```python
from build123d import *

# Parameters (mm, degrees)
SKETCH1_W                = 50
SKETCH1_H                = 40
BOSS_EXTRUDE1_DEPTH      = 20
SKETCH2_W                = 36
SKETCH2_H                = 16
CUT_EXTRUDE1_DEPTH       = 50
CUT_EXTRUDE2_REACH       = 53.235
BOSS_EXTRUDE2_DEPTH      = 5
BOSS_EXTRUDE2_DEPTH_BACK = 25
SKETCH5_R                = 9
BOSS_EXTRUDE3_START      = -19
SKETCH8_R                = 9
BOSS_EXTRUDE3_DEPTH      = 19
SKETCH9_R                = 8
CUT_EXTRUDE4_DEPTH       = 30


with BuildPart() as part:
    # Sketch1 → Boss-Extrude1 (new body)
    with BuildSketch(Plane(origin=(0, 0, 0), x_dir=(1, 0, 0), z_dir=(0, 1, 0))):
        Rectangle(SKETCH1_W, SKETCH1_H)
    extrude(amount=BOSS_EXTRUDE1_DEPTH)

    # Sketch2 → Cut-Extrude1 (cut)
    with BuildSketch(Plane(origin=(25, 0, 0), x_dir=(0, 0, -1), z_dir=(1, 0, 0))):
        with Locations((0, 10)):
            Rectangle(SKETCH2_W, SKETCH2_H)
    extrude(amount=-CUT_EXTRUDE1_DEPTH, mode=Mode.SUBTRACT)

    # Cut-Extrude2: up to this face of the body (flat: up to its plane)
    cut_extrude2_end = Plane(part.part.faces().sort_by_distance((0, 10, -20))[0])
    # Sketch3 → Cut-Extrude2 (cut, up to the picked face)
    with BuildSketch(Plane.XY.offset(20), mode=Mode.PRIVATE) as cut_extrude2_sk1:
        Polygon((25, 0), (25, 20), (10, 0), align=None)
    cut_extrude2_tool1 = split(extrude(cut_extrude2_sk1.sketch, amount=-CUT_EXTRUDE2_REACH, mode=Mode.PRIVATE), bisect_by=cut_extrude2_end, keep=Keep.BOTH, mode=Mode.PRIVATE)
    # Sketch3 → Cut-Extrude2 (cut, up to the picked face)
    with BuildSketch(Plane.XY.offset(20), mode=Mode.PRIVATE) as cut_extrude2_sk2:
        Polygon((-10, 0), (-25, 20), (-25, 0), align=None)
    cut_extrude2_tool2 = split(extrude(cut_extrude2_sk2.sketch, amount=-CUT_EXTRUDE2_REACH, mode=Mode.PRIVATE), bisect_by=cut_extrude2_end, keep=Keep.BOTH, mode=Mode.PRIVATE)
    add(cut_extrude2_tool1.solids().sort_by(Axis((20, 6.666667, 20), (0, 0, -1)))[0], mode=Mode.SUBTRACT)
    add(cut_extrude2_tool2.solids().sort_by(Axis((-20, 6.666667, 20), (0, 0, -1)))[0], mode=Mode.SUBTRACT)

    # Sketch5 → Boss-Extrude2 (add, two sides: drawn at the far end of the back side and taken through both)
    with BuildSketch(Plane(origin=(0, 20, 0), x_dir=(1, 0, 0), z_dir=(0, 1, 0)).offset(-BOSS_EXTRUDE2_DEPTH_BACK)):
        with Locations(Location((0, 0, 0), (0, 0, 90))):
            Circle(SKETCH5_R)
    extrude(amount=BOSS_EXTRUDE2_DEPTH + BOSS_EXTRUDE2_DEPTH_BACK)

    # Sketch8 → Boss-Extrude3 (add)
    with BuildSketch(Plane(origin=(0, -5, 0), x_dir=(-1, 0, 0), z_dir=(0, -1, 0)).offset(BOSS_EXTRUDE3_START)):
        with Locations(Location((0, 0, 0), (0, 0, 90))):
            Circle(SKETCH8_R)
    extrude(amount=BOSS_EXTRUDE3_DEPTH)

    # Sketch9 → Cut-Extrude4 (cut)
    with BuildSketch(Plane(origin=(0, 25, 0), x_dir=(1, 0, 0), z_dir=(0, 1, 0))):
        with Locations(Location((0, 0, 0), (0, 0, 270))):
            Circle(SKETCH9_R)
    extrude(amount=-CUT_EXTRUDE4_DEPTH, mode=Mode.SUBTRACT)


solid = part.part
```
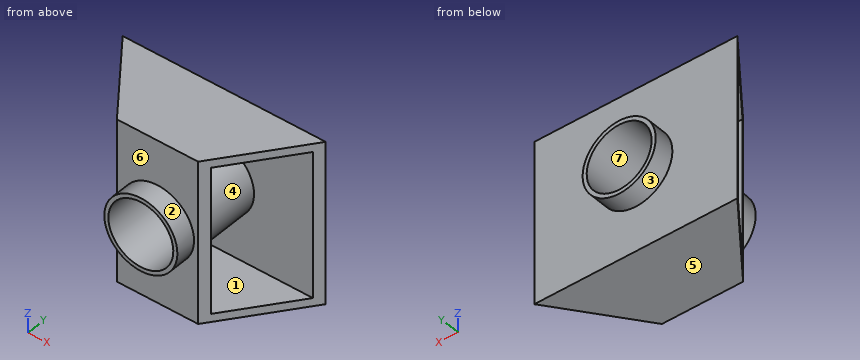
CAD build for the part. Positions are in the model's coordinates, mm. Face numbers are marked on the shaded views. A direction names the side the tool comes from. Coordinates: 2 decimals unless noted, no trailing zeros. Write each loop counter-clockwise with the first axis right and the second up, starting at its lowest first coordinate (ties: lowest second). Pieces come first, ordered by that corner, then holes. Notation, with made-up numbers: (13, -15) -> (72, -15) arc R9 cw to (72, -7) -> close; hole circle Ø2 at (-37, 4.5). An arc over 180 degrees is marked (long way). Use CSV: the item, a comma, the result in double quotes. Start each with the question number.
Item 1: Band-saw the part on B-B, the plane y = 11.25. Write the cut outline in (x, z).
Item 2: Two-plate mould, pull along Z, no slides. Class the marked faces 4, 5, 6 and 7: +Z half, -Z half, draft (parallel to the pull), parting line (faces both ways), or undercut.
Item 3: Band-saw the part on C-C, the plane z = 13.5. Write the cut outline in (x, y), plus the area to 3 significant figures.
Item 4: Band-saw the part on D-D, the plane y = 22.25. Write the cut outline in (x, z).
Item 5: Tool access for the marked faces 1, 2 and 3: list every direction of +Z, -Z, +X, -X, +Y, -Y with a clear straight run to the whole face (end or side of a thin tool).
Item 6: Band-saw the part on A-A, the plane x = 0. Write the cut outline in (y, z).
Item 7: Wall check: probe 1 along Y at (x, z) = (3.5, 11); probe 2 along Z at (x, y) = (-3, 6.25); probe 3 along Z at (x, y) = (-16.5, 11). Give the ranges that are in metal, low to high.
Item 8: Drop flat-ended pins along their axis: P1, Ø6, axis at y = 8.5, z = 1, coming from the -X side; P2, Ø1, axis at x = -16, z = 8, coming from the +Y side; P3, Ø13, axis at x = 0, z = 0, coming from the -Y side; P4, Ø6, axis at y = 15.5, z = 1.5, coming from the -X side (3 decimals). Give the stop position or say it passes through.
Response values:
1,outline,"(-18.44, -20) -> (18.44, -20) -> (18.44, -18) -> (-18.44, -18) -> close; (-18.44, 18) -> (18.44, 18) -> (18.44, 20) -> (-18.44, 20) -> close; circle Ø18 at (0, 0); hole circle Ø16 at (0, 0)"
2,face 4,"undercut"
2,face 5,"-Z half"
2,face 6,"draft"
2,face 7,"undercut"
3,outline,"(-25, 20) -> (-23.5, 18) -> (23.5, 18) -> (25, 20) -> close; (-11.5, 2) -> (-10, 0) -> (10, 0) -> (11.5, 2) -> close"
3,area,"140 mm2"
4,outline,"circle Ø18 at (0, 0); hole circle Ø16 at (0, 0)"
5,face 1,"+X, -X"
5,face 2,"-Y"
5,face 3,"+Y"
6,outline,"(-5, -9) -> (0, -9) -> (0, -20) -> (20, -20) -> (20, -9) -> (25, -9) -> (25, -8) -> (-5, -8) -> close; (-5, 8) -> (25, 8) -> (25, 9) -> (20, 9) -> (20, 20) -> (0, 20) -> (0, 9) -> (-5, 9) -> close; hole (2, -18) -> (18, -18) -> (18, -9) -> (2, -9) -> close; hole (2, 9) -> (18, 9) -> (18, 18) -> (2, 18) -> close"
7,probe 1,"y = 0 to 2, 18 to 20"
7,probe 2,"z = -20 to -18, -8.49 to -7.42, 7.42 to 8.49, 18 to 20"
7,probe 3,"z = -20 to -18, 18 to 20"
8,P1,"stops at x = -9"
8,P2,"stops at y = 20"
8,P3,"passes through"
8,P4,"stops at x = -23.875"
